Autodesk Inventor part; units mm, degrees
ref_plane "YZ Plane" through (0, 0, 0) normal (1, 0, 0) x (0, 1, 0)
ref_plane "XZ Plane" through (0, 0, 0) normal (0, 1, 0) x (-1, 0, 0)
ref_plane "XY Plane" through (0, 0, 0) normal (0, 0, 1) x (1, 0, 0)
sketch "Эскиз1" plane through (0, 0, 0) normal (0, 0, 1) x (1, 0, 0)
  line L0 (-88.2272, -119.1) -> (-57.3625, -234.2883)
  line L1 (-71.2043, -171.0391) -> (-83.11, -126.6066) construction
  line L2 (-69.083, -167.3649) -> (-79.4357, -128.7279)
  line L3 (-85.2313, -130.2808) -> (-74.8785, -168.9178)
  arc A0 (-74.8785, -168.9178) -> (-69.083, -167.3649) centre (-71.9807, -168.1414) ccw
  arc A1 (-79.4357, -128.7279) -> (-85.2313, -130.2808) centre (-82.3335, -129.5043) ccw
  line L4 (-68.8409, -165.5636) -> (-67.9892, -168.7423)
  line L5 (-67.9892, -168.7423) -> (-70.3162, -171.0693)
  line L6 (-70.3162, -171.0693) -> (-73.495, -170.2176)
  line L7 (-73.495, -170.2176) -> (-74.3467, -167.0388)
  line L8 (-74.3467, -167.0388) -> (-72.0197, -164.7118)
  line L9 (-72.0197, -164.7118) -> (-68.8409, -165.5636)
  line L10 (-72.3186, -163.5965) -> (-75.4621, -166.74)
  line L11 (-75.4621, -166.74) -> (-74.3115, -171.0341)
  line L12 (-74.3115, -171.0341) -> (-70.0173, -172.1847)
  line L13 (-70.0173, -172.1847) -> (-66.8738, -169.0412)
  line L14 (-66.8738, -169.0412) -> (-68.0244, -164.7471)
  line L15 (-68.0244, -164.7471) -> (-72.3186, -163.5965)
  line L16 (-77.1571, -148.8229) -> (-74.2593, -148.0464)
  line L17 (-78.3254, -130.1669) -> (-79.1772, -126.9881)
  line L18 (-79.1772, -126.9881) -> (-82.356, -126.1364)
  line L19 (-82.356, -126.1364) -> (-84.683, -128.4634)
  line L20 (-84.683, -128.4634) -> (-83.8312, -131.6422)
  line L21 (-80.6525, -132.4939) -> (-78.3254, -130.1669)
  line L22 (-80.3536, -133.6093) -> (-84.6477, -132.4587)
  line L23 (-85.7983, -128.1645) -> (-82.6548, -125.021)
  line L24 (-82.6548, -125.021) -> (-78.3607, -126.1716)
  line L25 (-78.3607, -126.1716) -> (-77.2101, -130.4657)
  line L26 (-77.2101, -130.4657) -> (-80.3536, -133.6093)
  line L27 (-83.8312, -131.6422) -> (-80.6525, -132.4939)
  point P0 (0, 0)
  point P1 (-71.168, -167.8906)
  point P2 (-69.9205, -164.239)
  point P3 (-78.5981, -131.8538)
  dimension "d0" = 0
  dimension "d2" = 40
  dimension "d3" = 3
  dimension "d4" = 5.7
  dimension "d5" = 1
  dimension "d6" = 1
extrude "Выдавливание1" add sketch "Эскиз1" along normal blind 2 contours L23 L24 L25 L26 L2 L21 L17 L18 L19 A1 L0 | A1 L19 L20 L27 L21 L2 L26 L22 L0 | L22 L26 L2 L15 L10 L0 | L10 L15 L2 L9 L8 L7 L6 A0 L0 | A0 L6 L5 L4 L9 L2 L15 L14 L13 L12 L0
sketch "Эскиз2" plane through (0, 0, 0) normal (0, 0, -1) x (-1, 0, 0)
  line L0 (78.3254, -130.1669) -> (80.6525, -132.4939)
  line L1 (84.683, -128.4634) -> (82.356, -126.1364)
  line L2 (83.8312, -131.6422) -> (84.683, -128.4634)
  line L3 (80.6525, -132.4939) -> (83.8312, -131.6422)
  line L4 (82.356, -126.1364) -> (79.1772, -126.9881)
  line L5 (79.1772, -126.9881) -> (78.3254, -130.1669)
  arc A0 (19.276, -252.9141) -> (17.0616, -251.2452) centre (19.4208, -250.4183) ccw
  arc A1 (19.276, -252.9141) -> (27.7531, -256.792) centre (35, -229.7461) ccw
  line L6 (48.5053, -262.3526) -> (27.7531, -256.792)
  line L7 (49.9977, -260.8602) -> (48.5053, -262.3526)
  arc A2 (51.783, -259.0748) -> (49.9977, -260.8602) centre (49.3645, -258.4417) ccw
  line L8 (60, -250.8579) -> (51.783, -259.0748)
  line L9 (60, -250.8579) -> (60, -245)
  line L10 (61.2941, -235.1704) -> (60, -245)
  line L11 (61.2941, -235.1704) -> (85, -146.6987)
  line L12 (85, -129.4867) -> (85, -146.6987)
  arc A3 (85, -111.5505) -> (85, -116.4495) centre (82.5, -114) ccw
  line L13 (85, -46.4495) -> (85, -111.5505)
  arc A4 (85, -41.5505) -> (85, -46.4495) centre (82.5, -44) ccw
  line L14 (85, -37.8284) -> (85, -41.5505)
  line L15 (76.4668, -29.2952) -> (85, -37.8284)
  arc A5 (72.9685, -21.4377) -> (76.4668, -29.2952) centre (84.9521, -20.8099) ccw
  arc A6 (72.9685, -21.4377) -> (27.398, -26.9013) centre (50, -22.641) ccw
  spline S0 degree 3 poles (27.6217, -27.9525) (27.5401, -27.6087) (27.4664, -27.263) (27.4007, -26.9157) (27.3998, -26.9109) (27.3989, -26.9061) (27.398, -26.9013) knots -4.945428 -4.945428 -4.945428 -4.945428 -4.899332 -4.899332 -4.899332 -4.898696 -4.898696 -4.898696 -4.898696 weights 1 1 1 1 1 1 1
  spline S1 degree 3 poles (28.164, -30.4631) (27.9989, -29.614) (27.8171, -28.7759) (27.6217, -27.9525) knots 3.015096 3.015096 3.015096 3.015096 3.260421 3.260421 3.260421 3.260421 weights 1 1 1 1
  spline S2 degree 3 poles (28.3854, -31.6677) (28.3156, -31.2645) (28.2417, -30.8629) (28.164, -30.4631) knots 1.901203 1.901203 1.901203 1.901203 2.021579 2.021579 2.021579 2.021579
  spline S3 degree 3 poles (27.2821, -32.2702) (27.4905, -32.4048) (27.7033, -32.5146) (27.9524, -32.5655) (28.0203, -32.5713) (28.1301, -32.5543) (28.1726, -32.54) (28.2472, -32.4946) (28.2776, -32.4662) (28.335, -32.3905) (28.358, -32.3417) (28.403, -32.2042) (28.4139, -32.1072) (28.4174, -31.9004) (28.4051, -31.7812) (28.3854, -31.6677) knots 0 0 0 0 0.074448 0.074448 0.10037 0.10037 0.118258 0.118258 0.134856 0.134856 0.155747 0.155747 0.191916 0.191916 0.237121 0.237121 0.237121 0.237121
  arc A7 (27.2821, -32.2702) -> (27.8696, -42.0032) centre (24, -37.3526) ccw
  spline S4 degree 3 poles (29.1017, -42.1691) (29.109, -42.0304) (29.1004, -41.9076) (29.061, -41.7446) (29.038, -41.6821) (28.9802, -41.5961) (28.9528, -41.5669) (28.8903, -41.5252) (28.8586, -41.5123) (28.7851, -41.4972) (28.7445, -41.4975) (28.6379, -41.5118) (28.5702, -41.5357) (28.3843, -41.6196) (28.2441, -41.7105) (28.0145, -41.8847) (27.9405, -41.9442) (27.8696, -42.0032) knots 0 0 0 0 0.041653 0.041653 0.066962 0.066962 0.083043 0.083043 0.096975 0.096975 0.113046 0.113046 0.139961 0.139961 0.194848 0.194848 0.220751 0.220751 0.220751 0.220751
  spline S5 degree 3 poles (28.9908, -43.6688) (28.9918, -43.6586) (28.9927, -43.6484) (29.0398, -43.1514) (29.0756, -42.6615) (29.1017, -42.1691) knots 0.829158 0.829158 0.829158 0.829158 0.832223 0.832223 0.978679 0.978679 0.978679 0.978679
  spline S6 degree 3 poles (19.7401, -60.1945) (21.5778, -59.1335) (23.1611, -57.7343) (25.061, -55.3244) (25.591, -54.5234) (27.536, -51.066) (28.3761, -48.1601) (28.7981, -45.2696) (28.876, -44.7357) (28.9396, -44.2038) (28.9908, -43.6688) knots 0 0 0 0 0.557778 0.557778 0.815105 0.815105 1.63021 1.63021 1.63021 1.780759 1.780759 1.780759 1.780759 weights 1 1 1 1 1 1 1 1 1 1 1
  line L16 (19.7253, -60.203) -> (19.7401, -60.1945)
  line L17 (7, -67.55) -> (19.7253, -60.203)
  line L18 (7, -229.7461) -> (7, -67.55)
  arc A8 (7, -229.7461) -> (17.0616, -251.2452) centre (35, -229.7461) ccw
  circle A9 centre (27.4442, -220.4746) radius 2.5
  circle A10 centre (38.4044, -239.4581) radius 7.5
  circle A11 centre (24, -107.3526) radius 4
  circle A12 centre (34.7265, -68.7944) radius 1.5
  circle A13 centre (34.7265, -138.7944) radius 1.5
  circle A14 centre (34.7265, -208.7944) radius 1.5
  circle A15 centre (43.2836, -60.3339) radius 1.5
  circle A16 centre (43.2836, -200.3339) radius 1.5
  circle A17 centre (43.2836, -130.3339) radius 1.5
  circle A18 centre (30.7187, -204.3292) radius 1.5
  circle A19 centre (30.7187, -134.3292) radius 1.5
  circle A20 centre (30.7187, -64.3292) radius 1.5
  circle A21 centre (38.7342, -73.2595) radius 1.5
  circle A22 centre (38.7342, -143.2595) radius 1.5
  circle A23 centre (38.7342, -213.2595) radius 1.5
  circle A24 centre (26.7109, -199.864) radius 1.5
  circle A25 centre (26.7109, -129.864) radius 1.5
  circle A26 centre (26.7109, -59.864) radius 1.5
  circle A27 centre (50, -22.641) radius 6
  circle A28 centre (24, -37.3526) radius 4
  circle A29 centre (24, -177.3526) radius 4
  circle A30 centre (57.3879, -228.498) radius 2.5
  line L19 (74.3467, -167.0388) -> (72.0197, -164.7118)
  line L20 (73.495, -170.2176) -> (74.3467, -167.0388)
  line L21 (70.3162, -171.0693) -> (73.495, -170.2176)
  line L22 (67.9892, -168.7423) -> (70.3162, -171.0693)
  line L23 (68.8409, -165.5636) -> (67.9892, -168.7423)
  line L24 (72.0197, -164.7118) -> (68.8409, -165.5636)
  line L25 (80.6525, -132.4939) -> (83.8312, -131.6422)
  line L26 (79.1772, -126.9881) -> (78.3254, -130.1669)
  circle A31 centre (81.5042, -129.3151) radius 1.5
  circle A32 centre (71.168, -167.8906) radius 1.5
  arc A33 (85, -129.1436) -> (85, -129.4867) centre (81.5042, -129.3151) ccw
  line L27 (85, -116.4495) -> (85, -129.1436)
  circle A34 centre (71.168, -167.8906) radius 3.5
  point P0 (0, 0)
  dimension "d9" = 3
  dimension "d10" = 3
extrude "Выдавливание2" add sketch "Эскиз2" against normal blind 0.2 contours L5 L4 L1 L2 L3 L0 | L20 L21 L22 L23 L24 L19
fillet "Сопряжение1" radius 2 10 edges at (-78.5981, -131.8538, 1) (-69.9205, -164.239, 1) (-68.0244, -164.7471, 1) (-66.8738, -169.0412, 1) (-70.0173, -172.1847, 1) (-74.3115, -171.0341, 1) (-82.6548, -125.021, 1) (-85.7983, -128.1645, 1) (-78.3607, -126.1716, 1) (-77.2101, -130.4657, 1)
properties part number "РельсКрышки"
The model under review builds one solid part; all positions refer to its coordinate system, in mm. A direction names the side the tool comes from. Round coordinates to 2 decimals unless told otherwise and drop trailing zeros. Order: outer loops, then holes, each group sorted by start corner. A loop starts at its lowest first (then second) coordinate and runs counter-clockwise, first axis right, second up. Notation, with made-up numbers: M 89,-26 L 134,-26 A24 cw 134,-14 Z; hole C -34.75,-12 d1. An arc over 180 degrees is marked long. Use a Markdown table: item, result.
1) Consider section A-A (z = 1.5). Give the number of separate pieces and of enclosed holes in the cut face, then the cut area to 3 significant figures.
Report:
| item | result |
|---|---|
| separate pieces | 1 |
| enclosed holes | 2 |
| area | 243 mm^2 |
2) Consider section C-C (x = -75.25). Write out the cut boundary in (y, z), then the cut area to 3 significant figures.
Report:
| item | result |
|---|---|
| outline | M -167.53,0 L -144.35,0 L -144.35,2 L -167.53,2 Z |
| area | 46.4 mm^2 |
3) Tool access review of faces 1 (the face through (-67.448, -166.9, 0.986)), 2 (the face through (-82.264, -132.062, 1.087)): name each direction out of +Z, -Z, +X, -X, +Y, -Y from which nothing blocks a thin tool from reaching the whole face with its end or side.
Report:
| item | result |
|---|---|
| face 1 | +Z, -Z, +X, +Y |
| face 2 | +Z |
4) Wall thickness on line 1 along X through (y, z) = (-168, 1.9); line 2 along X through (y, z) = (-131.5, 0.55); line 3 along Y through (x, z) = (-69.5, 0.9): over which ranges is each line inside the solid? List them lowest first. Write a range as [from, to].
Report:
| item | result |
|---|---|
| line 1 | [-75.12, -74.09], [-68.19, -67.15] |
| line 2 | [-84.9, -83.87], [-79.66, -78.13] |
| line 3 | [-171.61, -170.25], [-165.39, -164.2] |
5) Draft analysis for pull direction Y (two halves, no side actions). For faces 3 (the face through (-78.57, -126.4, 1.01)), 4 (the face through (-80.74, -126.57, 1.09)), 5 (the face through (-72.2, -171.6, 1)), 6 (the face through (-77, -148, 2)), state which applies: released by +Y, released by -Y, zero draft, split by the parting line, or undercut.
Report:
| item | result |
|---|---|
| face 3 | released by +Y |
| face 4 | undercut |
| face 5 | released by -Y |
| face 6 | zero draft |
6) Insertion check: pin 1 (1 mm diameter, centred on x = -83.5, z = 1.5, fed in from +Y); pin 2 (3 mm diameter, centred on x = -71, y = -169, fed in from +Z); pin 3 (2.5 mm diameter, centred on x = -81.5, y = -129.32, fed in from +Z). Each pin has a flat end and moves straight along its axis. Give the tip position at first contact, or say it passes through.
Report:
| item | result |
|---|---|
| pin 1 | y = -125.49 |
| pin 2 | z = 0.2 |
| pin 3 | through |
7) Consider section B-B (y = -136). Write out the cut boundary in (x, z), then the cut area to 3 significant figures.
Report:
| item | result |
|---|---|
| outline | M -83.7,0 L -77.49,0 L -77.49,2 L -83.7,2 Z |
| area | 12.4 mm^2 |
